The drawing under review shows one solid part. Ordinate dimensions are in mm from its lowest x, y, z. A direction names the side the tool comes from. Give positions to 0.01 mm unless a question says otherwise; leave off trailing zeros. Order: outer loops, then holes, each group sorted by start corner. A loop starts at its lowest first (then second) coordinate and runs counter-clockwise, first axis right, second up. Notation, with made-up numbers: (36.5, 4.5) -> (50.5, 4.5) arc R11 ccw to (50.5, 18.5) -> close; hole circle Ø7 at (42.25, -12). An arc over 180 degrees is marked (long way). Use CSV: the item, a comma, the result in double quotes. Start each with the question number.
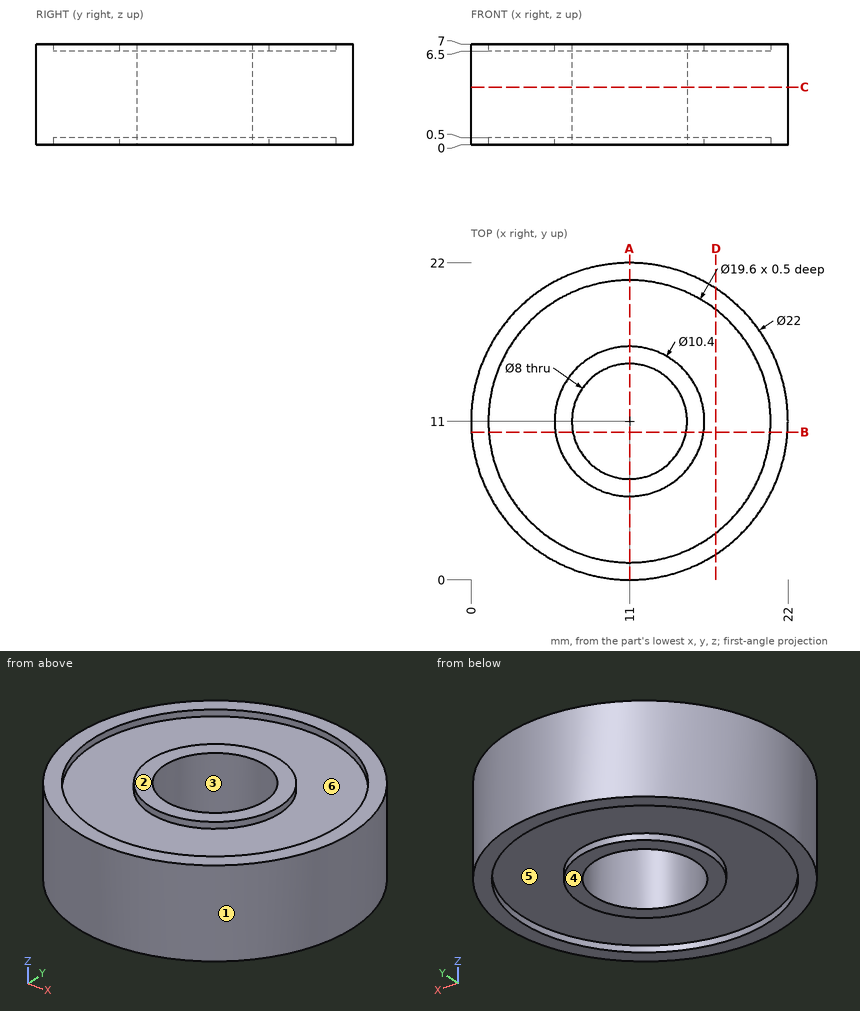
1. Consider section A-A (x = 11). State the section outline as (y, z) points.
2. To check wall thickness, follow L1, parallel to Y at x = 11, z = 6.75; L2, parallel to Y at x = 11, z = 4.75; L3, parallel to Z at x = 8.25, y = 16.5. State the ranges of each line that lie inside material, in increasing order. Write a range as [from, to].
3. Clearance check with a flat-ended pin moving along its axis: P1, Ø3, axis at x = 14.5, z = 2.5, coming from the +Y side. State where the tip first meets the part, or that it passes through.
4. Draft analysis for pull direction Y (two halves, no side actions). For the marked faces 1, 2 and 3, state which applies: +Y half, -Y half, draft (parallel to the pull), parting line (faces both ways), or undercut.
5. Consider section D-D (x = 17). State the section outline as (y, z) points.
6. For the marked faces 4, 5 and 6, list the 3-axis set-ups (+Z, -Z, +X, -X, +Y, -Y) from which the entire face can be reached by the end or side of a thin tool; tool diameter is ignored.
7. Consider section B-B (y = 10.25). State the section outline as (x, z) points, plus the area to 3 significant figures.
8. Consider section C-C (z = 4). State the section outline as (x, y) points, plus the area to 3 significant figures.
Answer list:
1,outline,"(0, 0) -> (1.2, 0) -> (1.2, 0.5) -> (5.8, 0.5) -> (5.8, 0) -> (7, 0) -> (7, 7) -> (5.8, 7) -> (5.8, 6.5) -> (1.2, 6.5) -> (1.2, 7) -> (0, 7) -> close; (15, 0) -> (16.2, 0) -> (16.2, 0.5) -> (20.8, 0.5) -> (20.8, 0) -> (22, 0) -> (22, 7) -> (20.8, 7) -> (20.8, 6.5) -> (16.2, 6.5) -> (16.2, 7) -> (15, 7) -> close"
2,L1,"[0, 1.2], [5.8, 7], [15, 16.2], [20.8, 22]"
2,L2,"[0, 7], [15, 22]"
2,L3,"[0.5, 6.5]"
3,P1,"y = 21.82"
4,face 1,"parting line"
4,face 2,"draft"
4,face 3,"undercut"
5,outline,"(1.78, 0) -> (3.25, 0) -> (3.25, 0.5) -> (18.75, 0.5) -> (18.75, 0) -> (20.22, 0) -> (20.22, 7) -> (18.75, 7) -> (18.75, 6.5) -> (3.25, 6.5) -> (3.25, 7) -> (1.78, 7) -> close"
6,face 4,"-Z, +X, -X, +Y, -Y"
6,face 5,"-Z"
6,face 6,"+Z"
7,outline,"(0.03, 0) -> (1.23, 0) -> (1.23, 0.5) -> (5.85, 0.5) -> (5.85, 0) -> (7.07, 0) -> (7.07, 7) -> (5.85, 7) -> (5.85, 6.5) -> (1.23, 6.5) -> (1.23, 7) -> (0.03, 7) -> close; (14.93, 0) -> (16.15, 0) -> (16.15, 0.5) -> (20.77, 0.5) -> (20.77, 0) -> (21.97, 0) -> (21.97, 7) -> (20.77, 7) -> (20.77, 6.5) -> (16.15, 6.5) -> (16.15, 7) -> (14.93, 7) -> close"
7,area,"89.4 mm2"
8,outline,"circle Ø22 at (11, 11); hole circle Ø8 at (11, 11)"
8,area,"330 mm2"
